from build123d import *

# Parameters (mm, degrees)
BOSS_EXTRUDE1_DEPTH      = 150
BOSS_EXTRUDE1_DEPTH_BACK = 68
SKETCH2_R                = 100
CUT_EXTRUDE1_DEPTH       = 20
CUT_EXTRUDE1_DEPTH_BACK  = 200
SKETCH6_R                = 90
FILLET1_R                = 10


with BuildPart() as part:
    # Sketch2 → Boss-Extrude1 (new, two sides: drawn at the far end of the back side and taken through both)
    with BuildSketch(Plane.XY.offset(-BOSS_EXTRUDE1_DEPTH_BACK)):
        Circle(SKETCH2_R)
    extrude(amount=BOSS_EXTRUDE1_DEPTH + BOSS_EXTRUDE1_DEPTH_BACK)

    # Sketch6 → Cut-Extrude1 (cut, two sides: drawn at the far end of the back side and taken through both)
    with BuildSketch(Plane(origin=(0, 0, -68), x_dir=(-1, 0, 0), z_dir=(0, 0, -1)).offset(-CUT_EXTRUDE1_DEPTH_BACK)):
        with Locations(Location((0, 0, 0), (0, 0, 180))):
            Circle(SKETCH6_R)
    extrude(amount=CUT_EXTRUDE1_DEPTH + CUT_EXTRUDE1_DEPTH_BACK, mode=Mode.SUBTRACT)

    # Fillet1
    fillet1_edges = [part.edges().sort_by_distance(p)[0] for p in [
        (-100, 0, 150),
    ]]
    fillet(fillet1_edges, radius=FILLET1_R)


solid = part.part
Geometry: final body of the model. Coordinates: model frame, mm. A direction names the side the tool comes from. Coordinates: 2 decimals unless noted, no trailing zeros. Order: outer loops, then holes, each group sorted by start corner. A loop starts at its lowest first (then second) coordinate and runs counter-clockwise, first axis right, second up. Notation, with made-up numbers: (33, 54) - (51, 54) arc R25 cw to (51, 90) - close; hole circle Ø6 at (4, -14.5). An arc over 180 degrees is marked (long way). Use one line per item in the form item = value.
1) Mould query, pull axis X, two halves, no side actions, for faces 1 (the face through (-1, 1, 150)), 2 (the face through (95.38, 30.04, 34.54)), 3 (the face through (41.53, 79.845, 33.4)). Classes: +X half, -X half, draft (parallel to the pull), parting line (faces both ways), or undercut.
Solutions:
face_1 = draft
face_2 = parting line
face_3 = undercut
2) Pin query (flat end, axial travel): pin 1 (8 mm diameter, centred on x = -25.5, z = 20, fed in from -Y); pin 2 (12 mm diameter, centred on x = 75.5, y = -77, fed in from +Z); pin 3 (8 mm diameter, centred on x = 49.5, z = 121, fed in from +Y); pin 4 (1 mm diameter, centred on y = 25, z = 3.5, fed in from -X). Return the tip coordinate at first contact, or that it passes through.
Solutions:
pin_1 = -97.66
pin_2 = through
pin_3 = 89.05
pin_4 = -96.95
3) Ray query, L1, parallel to Y at x = 0, z = 66; L2, parallel to Z at x = 10, y = 75.5; L3, parallel to Y at x = 53.5, z = 115. Return the intervals inside material, ascending.
Solutions:
L1 = -100 to -90, 90 to 100
L2 = 132 to 150
L3 = -84.49 to -72.37, 72.37 to 84.49
4) Section B-B (y = 0). Return loops of the section in (x, z).
Solutions:
outline = (-100, -68) - (-90, -68) - (-90, 132) - (90, 132) - (90, -68) - (100, -68) - (100, 140) arc R10 ccw to (90, 150) - (-90, 150) arc R10 ccw to (-100, 140) - close
5) Set-up query: faces 4 (the face through (-82, 38, -68)), 5 (the face through (-1, -1, 132)). Return all of +Z, -Z, +X, -X, +Y, -Y with unobstructed straight access to the full face (end or side cutting, diameter ignored); none if empty.
Solutions:
face_4 = -Z, +X, -X, +Y, -Y
face_5 = -Z
6) Section A-A (z = 101.5). Return loops of the section in (x, y), then the cut area to 3 significant figures.
Solutions:
outline = circle Ø200 at (0, 0); hole circle Ø180 at (0, 0)
area = 5,970 mm^2
